For this review, take the finished solid that the model builds, in its own axes (mm). A direction names the side the tool comes from. Give positions to 0.01 mm unless a question says otherwise; leave off trailing zeros. Write each loop counter-clockwise with the first axis right and the second up, starting at its lowest first coordinate (ties: lowest second). Pieces come first, ordered by that corner, then holes.
1) For P1, Ø1.2, axis at x = 50.5, z = 1, coming from the +Y side; P2, Ø2, axis at x = -85, z = 1.5, coming from the +Y side; P3, Ø0.5, axis at x = -127.5, z = 2, coming from the -Y side (3 decimals), all flat-tipped, find the tip position at first contact; note any pin that passes through.
2) Machinability: for faces 4 (the face through (110, 15, 2)), 5 (the face through (122, 1, 2)), 6 (the face through (9.76, 9.12, 2.03)), 7 (the face through (55, -9, 2)), which of the approach directions +Z, -Z, +X, -X, +Y, -Y give a long, thin tool a straight path to every point of the face, cutting with its end or side? Answer none if there is none.
3) Draft analysis for pull direction X (two halves, no side actions). For faces 1 (the face through (10.26, 5.14, 2.03)), 2 (the face through (-130, -6, 2)), 3 (the face through (120, 16.5, 2)), state which applies: pulls with the +X half, pulls with the -X half, needs draft (parallel to the pull), parting line crosses it, or undercut.
4) We need section A-A on z = 2.35. Give the number of separate pieces and of enclosed holes in the cut face, and give its area (3 significant figures).
5) Wall thickness on line 1 along Y through (x, z) = (51, 2.3); line 2 along X through (y, z) = (1, 1.4); line 3 along Y through (x, z) = (3.5, 2.4): over which ranges is each line inside the solid? List them lowest first.
6) We need section B-B on x = -9. Give the boundary of the cut face in (y, z), and give its area (3 significant figures).
Autodesk Inventor part; units mm, degrees
ref_plane "YZ Plane" through (0, 0, 0) normal (1, 0, 0) x (0, 1, 0)
ref_plane "XZ Plane" through (0, 0, 0) normal (0, 1, 0) x (-1, 0, 0)
ref_plane "XY Plane" through (0, 0, 0) normal (0, 0, 1) x (1, 0, 0)
sketch "Sketch1" plane through (0, 0, 0) normal (0, 0, 1) x (1, 0, 0)
  line L0 (-130, 16.5) -> (130, 16.5)
  line L1 (130, 16.5) -> (130, -16.5)
  line L2 (130, -16.5) -> (-130, -16.5)
  line L3 (-130, -16.5) -> (-130, 16.5)
  point P0 (0, 0)
  dimension "d0" = 260
  dimension "d1" = 33
  dimension "d2" = 16.5
  dimension "d3" = 130
extrude "Base" add sketch "Sketch1" along normal blind 4
sketch "Sketch2" plane through (0, 0, 4) normal (0, 0, 1) x (1, 0, 0)
  line L0 (130, 16.5) -> (130, -16.5)
  line L1 (-130, 16.5) -> (130, 16.5)
  line L2 (-130, -16.5) -> (-130, 16.5)
  line L3 (130, -16.5) -> (-130, -16.5)
  line L4 (75, 16.5) -> (110, 16.5)
  line L5 (110, 16.5) -> (110, 12.5)
  line L6 (110, 12.5) -> (75, 12.5)
  line L7 (75, 12.5) -> (75, 16.5)
  line L8 (-130, 16.5) -> (55, 16.5)
  line L9 (55, 16.5) -> (55, 12.5)
  line L10 (55, 12.5) -> (-130, 12.5)
  line L11 (-130, 12.5) -> (-130, 16.5)
  line L12 (35, -7.5) -> (55, -7.5)
  line L13 (55, -7.5) -> (55, -16.5)
  line L14 (55, -16.5) -> (35, -16.5)
  line L15 (35, -16.5) -> (35, -7.5)
  line L16 (75, -7.5) -> (110, -7.5)
  line L17 (110, -7.5) -> (110, -16.5)
  line L18 (110, -16.5) -> (75, -16.5)
  line L19 (75, -16.5) -> (75, -7.5)
  line L20 (110, -11.5) -> (130, -11.5)
  line L21 (130, -11.5) -> (130, -16.5)
  line L22 (130, -16.5) -> (110, -16.5)
  line L23 (110, -16.5) -> (110, -11.5)
  line L24 (55, -11.5) -> (75, -11.5)
  line L25 (75, -11.5) -> (75, -16.5)
  line L26 (75, -16.5) -> (55, -16.5)
  line L27 (55, -16.5) -> (55, -11.5)
  point P0 (0, 0)
  dimension "d6" = 35
  dimension "d7" = 4
  dimension "d8" = 0
  dimension "d9" = 20
  dimension "d10" = 185
  dimension "d11" = 4
  dimension "d12" = 0
  dimension "d13" = 0
  dimension "d14" = 20
  dimension "d15" = 20
  dimension "d16" = 9
  dimension "d17" = 0
  dimension "d18" = 165
  dimension "d19" = 35
  dimension "d20" = 9
  dimension "d21" = 0
  dimension "d22" = 20
  dimension "d23" = 20
  dimension "d24" = 5
  dimension "d25" = 20
  dimension "d26" = 5
  dimension "d27" = 0
  dimension "d28" = 0
  dimension "d29" = 0
  dimension "d30" = 0
  dimension "d98" = 20
extrude "StructureMounting" cut sketch "Sketch2" against normal blind 4 contours L0 L3 L17 L20 | L5 L6 L7 L1 | L17 L3 L19 L16 | L9 L10 L2 L1 | L3 L13 L24 L19 | L3 L15 L12 L13
sketch "Sketch4" plane through (0, 0, 4) normal (0, 0, 1) x (1, 0, 0)
  line L0 (55, 12.5) -> (-130, 12.5)
  line L1 (-130, -16.5) -> (-130, 12.5)
  line L2 (35, -16.5) -> (-130, -16.5)
  line L3 (35, -16.5) -> (35, -7.5)
  line L4 (55, 16.5) -> (55, 12.5)
  line L5 (35, -7.5) -> (-130, -16.5)
  line L6 (-130, 3.5) -> (35, 12.5)
  point P0 (0, 0)
  dimension "d42" = 20
  dimension "d43" = 20
extrude "MotorRamp" cut sketch "Sketch4" against normal blind 4
sketch "Sketch5" plane through (0, 0, 4) normal (0, 0, 1) x (1, 0, 0)
  line L0 (110, 12.5) -> (75, 12.5)
  line L1 (75, 12.5) -> (75, 16.5)
  line L2 (94.274, 12.5) -> (98.274, 12.5)
  line L3 (98.274, 12.5) -> (98.274, 2.5)
  line L4 (98.274, 2.5) -> (94.274, 2.5)
  line L5 (94.274, 2.5) -> (94.274, 12.5)
  line L6 (110, 16.5) -> (110, 12.5)
  point P0 (0, 0)
  dimension "d46" = 4
  dimension "d47" = 10
  dimension "d48" = 0
  dimension "d49" = 19.274
  dimension "d100" = 11.726
extrude "LowSleeve" [suppressed]
sketch "Sketch6" plane through (0, 0, 4) normal (0, 0, 1) x (1, 0, 0)
  line L0 (-130, -16.5) -> (-130, 3.5)
  line L1 (-120, -2.5) -> (-105, -2.5)
  line L2 (-105, -2.5) -> (-105, -6.5)
  line L3 (-105, -6.5) -> (-120, -6.5)
  line L4 (-120, -6.5) -> (-120, -2.5)
  line L5 (-90, -2.5) -> (-75, -2.5)
  line L6 (-75, -2.5) -> (-75, -6.5)
  line L7 (-75, -6.5) -> (-90, -6.5)
  line L8 (-90, -6.5) -> (-90, -2.5)
  line L9 (98.274, 2.5) -> (94.274, 2.5)
  line L10 (-106.4171, -4.5) -> (-87.4505, -4.5) construction
  circle A0 centre (-97.5, -4.5) radius 1.25
  point P0 (0, 0)
  dimension "d63" = 15
  dimension "d64" = 4
  dimension "d67" = 30
  dimension "d72" = 10
  dimension "d73" = 10
  dimension "d166" = 2
  dimension "d167" = 2.5
  dimension "d168" = 7.5
extrude "MotorSleeves" cut sketch "Sketch6" against normal blind 4
sketch "Sketch10" plane through (0, 0, 4) normal (0, 0, 1) x (1, 0, 0)
  line L0 (130, 16.5) -> (130, -11.5)
  line L1 (122, 6) -> (130, 6)
  line L2 (130, 6) -> (130, -4)
  line L3 (130, -4) -> (122, -4)
  line L4 (122, -4) -> (122, 6)
  point P0 (0, 0)
  dimension "d109" = 8
  dimension "d110" = 10
  dimension "d111" = 0
  dimension "d112" = 4
extrude "Cabling" cut sketch "Sketch10" against normal blind 4
sketch "Sketch12" plane through (0, 0, 4) normal (0, 0, 1) x (1, 0, 0)
  line L0 (35, 12.5) -> (-130, 3.5)
  line L1 (-0.084, 8.5834) -> (19.8863, 9.6726)
  line L2 (19.8863, 9.6726) -> (20.1041, 5.6786)
  line L3 (20.1041, 5.6786) -> (0.1338, 4.5893)
  line L4 (0.1338, 4.5893) -> (-0.084, 8.5834)
  point P0 (0, 0)
  dimension "d124" = 4
  dimension "d125" = 20
  dimension "d126" = 2
  dimension "d127" = 130
extrude "ESCholder" cut sketch "Sketch12" against normal blind 4
sketch "Sketch13" plane through (0, 0, 4) normal (0, 0, 1) x (1, 0, 0)
  line L0 (55, 16.5) -> (55, 12.5)
  line L1 (55, 12.5) -> (35, 12.5)
  line L2 (35, 12.5) -> (-130, 3.5)
  line L3 (-130, -16.5) -> (35, -7.5)
  line L4 (-30.0123, 6.4502) -> (-26.0182, 6.668)
  line L5 (-26.0182, 6.668) -> (-25.7459, 1.6754)
  line L6 (-25.7459, 1.6754) -> (-29.7399, 1.4576)
  line L7 (-29.7399, 1.4576) -> (-30.0123, 6.4502)
  line L8 (-47.5366, -2.0169) -> (-6.9954, 0.1945) construction
  line L9 (-29.1953, -8.5276) -> (-25.2012, -8.3097)
  line L10 (-25.2012, -8.3097) -> (-25.4736, -3.3171)
  line L11 (-25.4736, -3.3171) -> (-29.4676, -3.535)
  line L12 (-29.4676, -3.535) -> (-29.1953, -8.5276)
  line L13 (20.1041, 5.6786) -> (0.1338, 4.5893)
  line L14 (-27.9377, 5.1382) -> (-27.2725, -7.0585) construction
  circle A0 centre (-27.6051, -0.9601) radius 1.25
  line L15 (49, 10) -> (53, 10)
  line L16 (53, 10) -> (53, 5)
  line L17 (53, 5) -> (49, 5)
  line L18 (49, 5) -> (49, 10)
  line L19 (39.5253, 2.5) -> (63.8345, 2.5) construction
  line L20 (49, -5) -> (53, -5)
  line L21 (53, -5) -> (53, 0)
  line L22 (53, 0) -> (49, 0)
  line L23 (49, 0) -> (49, -5)
  circle A1 centre (51, 2.5) radius 1.25
  point P0 (0, 0)
  dimension "d134" = 2.5
  dimension "d135" = 7.5
  dimension "d136" = 4
  dimension "d137" = 100
  dimension "d140" = 10
  dimension "d151" = 2
  dimension "d152" = 2.5
  dimension "d153" = 4
  dimension "d154" = 5
  dimension "d155" = 2.5
  dimension "d156" = 6
  dimension "d157" = 10
  dimension "d158" = 2.5
  dimension "d159" = 2
extrude "CrossSupports" cut sketch "Sketch13" against normal blind 10
sketch "Sketch14" plane through (0, 0, 4) normal (0, 0, 1) x (1, 0, 0)
  line L0 (110, 12.5) -> (75, 12.5)
  circle A0 centre (113, 8) radius 3
  circle A1 centre (105, 8) radius 3
  point P0 (98.274, 12.5)
  point P1 (0, 0)
  dimension "d141" = 6
  dimension "d142" = 6
  dimension "d143" = 4.5
  dimension "d144" = 4.5
  dimension "d145" = 3
  dimension "d146" = 8
extrude "ESCpowerHoles" [suppressed]
sketch "Sketch15" plane through (0, 0, 4) normal (0, 0, 1) x (1, 0, 0)
  line L0 (75, -7.5) -> (110, -7.5)
  line L1 (94.274, 2.5) -> (98.274, 2.5)
  line L2 (98.274, 2.5) -> (98.274, -7.5)
  line L3 (98.274, -7.5) -> (94.274, -7.5)
  line L4 (94.274, -7.5) -> (94.274, 2.5)
  point P0 (0, 0)
extrude "HighSleeve" cut sketch "Sketch15" against normal blind 10
sketch "Sketch16" plane through (0, 0, 4) normal (0, 0, 1) x (1, 0, 0)
  line L0 (-130, -16.5) -> (-130, 3.5)
  line L1 (-128, 1.5) -> (-126.4, 1.5)
  line L2 (-126.4, 1.5) -> (-126.4, -13.5)
  line L3 (-126.4, -13.5) -> (-128, -13.5)
  line L4 (-128, -13.5) -> (-128, 1.5)
  point P0 (0, 0)
  dimension "d160" = 1.6
  dimension "d161" = 15
  dimension "d162" = 2
  dimension "d163" = 2
extrude "WingLedCutout" cut sketch "Sketch16" against normal blind 10
fillet "ImpactReduction" radius 5 2 edges at (-130, 3.5, 2) (-130, -16.5, 2)
properties part number "ArmInsideHigh"
Results list:
1. P1: stops at y = 12.5
1. P2: stops at y = 6.01
1. P3: stops at y = -15.685
2. face 4: +Z, -Z, +Y
2. face 5: +Z, -Z, +X
2. face 6: +Z, -Z
2. face 7: +Z, -Z, -Y
3. face 1: undercut
3. face 2: pulls with the -X half
3. face 3: needs draft
4. separate pieces: 1
4. enclosed holes: 11
4. area: 5,070 mm2
5. line 1: y = -7.5 to -5, 0 to 1.25, 3.75 to 5, 10 to 12.5
5. line 2: x = -129.47 to -128, -126.4 to 94.27, 98.27 to 122
5. line 3: y = -9.22 to 4.77, 8.78 to 10.78
6. outline: (-9.9, 0) - (10.1, 0) - (10.1, 4) - (-9.9, 4) - close
6. area: 80.0 mm2
